Autodesk Inventor part; units mm, degrees
ref_plane "YZ Plane" through (0, 0, 0) normal (1, 0, 0) x (0, 1, 0)
ref_plane "XZ Plane" through (0, 0, 0) normal (0, 1, 0) x (-1, 0, 0)
ref_plane "XY Plane" through (0, 0, 0) normal (0, 0, 1) x (1, 0, 0)
sketch "Sketch1" plane through (0, 0, 0) normal (0, 0, 1) x (1, 0, 0)
  line L0 (-48.5, 0) -> (-48.5, 55)
  line L1 (-48.5, 55) -> (-38.5, 55)
  line L2 (-38.5, 55) -> (-38.5, 27)
  line L3 (-30.5, 19) -> (30.5, 19)
  line L4 (38.5, 27) -> (38.5, 55)
  line L5 (38.5, 55) -> (48.5, 55)
  line L6 (48.5, 55) -> (48.5, 0)
  line L7 (48.5, 0) -> (-48.5, 0)
  arc A0 (-38.5, 27) -> (-30.5, 19) centre (-30.5, 27) ccw
  arc A1 (30.5, 19) -> (38.5, 27) centre (30.5, 27) ccw
  line L8 (0, 0) -> (0, 59.4805) construction
  point P0 (0, 0)
  point P1 (0, 19)
  dimension "d0" = 10
  dimension "d1" = 19
  dimension "d2" = 36
  dimension "d3" = 8
  dimension "d4" = 97
extrude "Extrusion1" add sketch "Sketch1" against normal blind 22
sketch "Sketch2" plane through (0, 0, 0) normal (0, 0, 1) x (1, 0, 0)
  arc A0 (24.6577, 0) -> (-24.6577, 0) centre (0, -34) ccw
  line L0 (-48.5, 0) -> (48.5, 0)
  line L1 (-24.6577, 0) -> (24.6577, 0)
  point P0 (0, 0)
  point P1 (0, 0)
  point P2 (0, 0)
  point P3 (-24.6577, 0)
  point P4 (24.6577, 0)
  dimension "d7" = 84
  dimension "d8" = 8
extrude "Extrusion2" cut sketch "Sketch2" against normal up to surface (22 mm away)
sketch "Sketch3" plane through (0, 0, 0) normal (0, 0, 1) x (1, 0, 0)
  arc A0 (24.6577, 0) -> (-24.6577, 0) centre (0, -34) ccw
  line L0 (-7, 7.4126) -> (-7, 13.4126)
  line L1 (-7, 13.4126) -> (7, 13.4126)
  line L2 (7, 13.4126) -> (7, 7.4126)
  line L3 (0, 0) -> (0, 19) construction
  line L4 (30.5, 19) -> (-30.5, 19)
  dimension "d11" = 14
  dimension "d12" = 6
extrude "Extrusion3" cut sketch "Sketch3" against normal up to surface (22 mm away)
sketch "Sketch4" plane through (0, 0, 0) normal (0, 0, 1) x (1, 0, 0)
  line L0 (-48.5, 55) -> (-48.5, 0)
  line L1 (-48.5, 0) -> (-24.6577, 0)
  point P0 (0, 0)
  point P1 (-36, 16)
  dimension "d22" = 12.5
  dimension "d23" = 16
hole "Hole1" at (-36, 16, 0) direction (0, 0, -1) diameter 5.5 depth 22
sketch "Sketch5" plane through (-48.5, 0, 0) normal (-1, 0, 0) x (0, 0, 1)
  line L0 (0, 55) -> (-22, 55)
  arc A0 (-17, 55) -> (-5, 55) centre (-11, 55) ccw
  line L1 (-17, 55) -> (-5, 55)
  point P0 (0, 0)
  point P1 (-5, 55)
  dimension "d24" = 12
extrude "Extrusion4" cut sketch "Sketch5" against normal up to surface (10 mm away)
mirror "Mirror1" about plane through (0, 0, 0) normal (1, 0, 0) of "Extrusion4"
sketch "Sketch6" plane through (-48.5, 55, 0) normal (0, 1, 0) x (1, 0, 0)
  line L0 (0, 5) -> (0, 17)
  line L1 (0, 22) -> (10, 22)
  point P0 (48.5, 0)
  point P1 (5, 19)
  point P2 (5, 3)
  point P3 (0, 11)
  point P4 (5, 22)
  dimension "d27" = 8
  dimension "d28" = 8
hole "Hole2" at (-43.5, 55, -19) at (-43.5, 55, -3) direction (0, -1, 0) diameter 3 depth 5
mirror "Mirror2" about plane through (0, 0, 0) normal (1, 0, 0) of "Hole2"
fillet "Fillet1" radius 8 2 edges at (48.5, 0, -11) (-48.5, 0, -11)
sketch "Sketch7" plane through (48.5, 55, -11) normal (1, 0, 0) x (0, 0, -1)
  line L0 (-11, -55) -> (11, -55)
  point P0 (0, -42)
  point P1 (0, -55)
  dimension "d44" = 13
hole "Hole3" at (48.5, 13, -11) direction (-1, 0, 0) diameter 3.242 depth 19
sketch "Sketch8" plane through (-30.5, 19, 0) normal (0, 1, 0) x (1, 0, 0)
  line L0 (-8, 17) -> (-8, 5)
  circle A0 centre (-13, 3) radius 1.5
  circle A1 centre (-13, 19) radius 1.5
  point P0 (30.5, 0)
  point P1 (30.5, 18)
  point P2 (30.5, 4)
  point P3 (-8, 11)
  dimension "d52" = 7
  dimension "d53" = 7
  dimension "d54" = 43.5
  dimension "d55" = 43.5
hole "Hole4" at (0, 19, -18) at (0, 19, -4) direction (0, -1, 0) diameter 4 end through all
sketch "Skizze9" plane through (0, 0, 0) normal (0, 0, 1) x (1, 0, 0)
  circle A0 centre (-36, 16) radius 2.75
  arc A1 (-48.5, 8) -> (-40.5, 0) centre (-40.5, 8) ccw
  line L0 (-40.5, 0) -> (-24.6577, 0)
  arc A2 (-7, 7.4126) -> (-24.6577, 0) centre (0, -34) ccw
  line L1 (-7, 7.4126) -> (-7, 13.4126)
  line L2 (-7, 13.4126) -> (7, 13.4126)
  line L3 (7, 13.4126) -> (7, 7.4126)
  arc A3 (24.6577, 0) -> (7, 7.4126) centre (0, -34) ccw
  line L4 (24.6577, 0) -> (40.5, 0)
  arc A4 (40.5, 0) -> (48.5, 8) centre (40.5, 8) ccw
  line L5 (48.5, 8) -> (48.5, 55)
  line L6 (48.5, 55) -> (38.5, 55)
  line L7 (38.5, 55) -> (38.5, 27)
  arc A5 (30.5, 19) -> (38.5, 27) centre (30.5, 27) ccw
  line L8 (30.5, 19) -> (-30.5, 19)
  arc A6 (-38.5, 27) -> (-30.5, 19) centre (-30.5, 27) ccw
  line L9 (-38.5, 27) -> (-38.5, 55)
  line L10 (-38.5, 55) -> (-48.5, 55)
  line L11 (-48.5, 55) -> (-48.5, 8)
  arc A7 (24.6577, 0) -> (-24.6577, 0) centre (0, -34) ccw
  point P0 (0, 0)
properties part number "145 part 2" material "Aluminum 6061-AHC"
CAD build for the part. Positions are in the model's coordinates, mm. A direction names the side the tool comes from. Coordinates: 2 decimals unless noted, no trailing zeros. Loops run counter-clockwise (first coordinate to the right, second up) from the corner with the lowest first, then second, coordinate; pieces in that order, holes last. Notation, with made-up numbers: (-27.5, 2) - (-11.5, 2) arc R24 cw to (-11.5, 41) - close; hole circle Ø10 at (61, -34.5). An arc over 180 degrees is marked (long way). Return JSON: item names as keys, results as strings.
1. Band-saw the part on C-C (y = 37). Give the cut face in (x, z), and give its area (3 significant figures).
Result:
{"outline": "(-48.5, -22) - (-38.5, -22) - (-38.5, 0) - (-48.5, 0) - close; (38.5, -22) - (48.5, -22) - (48.5, 0) - (38.5, 0) - close", "area": "440 mm2"}
2. 3-axis set-ups, long thin cutter, end or side, ignore diameter. For faces 1 (the flat face through (43, 55, -21)), 2 (the cylindrical face through (-16.13, 4.78, -10.85)), 3 (the cylindrical face through (38.87, 11.9, -9.81)), 4 (the flat face through (44, 50, -3)): which of +Z, -Z, +X, -X, +Y, -Y reach the whole face in a straight line?
Result:
{"face 1": "+Z, -Z, +X, -X, +Y", "face 2": "+Z, -Z, -Y", "face 3": "+X", "face 4": "+Y"}
3. Probe L1, parallel to X at y = 53.8, z = -3; L2, parallel to Z at x = 0, y = 16.6; L3, parallel to X at y = 44.5, z = -7.5. List the from-to ranges inside material, lowest first. Write a range as from..to.
Result:
{"L1": "x = -48.5..-45, -42..-38.5, 38.5..42, 45..48.5", "L2": "z = -22..-20, -16..-6, -2..0", "L3": "x = -48.5..-38.5, 38.5..48.5"}
4. Drop flat-ended pins along their axis: pin 1 (11 mm diameter, centred on x = 15, z = -12, fed in from +Y); pin 2 (4.5 mm diameter, centred on x = -36, y = 16, fed in from +Z); pin 3 (2.5 mm diameter, centred on x = 43.5, z = -3, fed in from -Y); pin 4 (11 mm diameter, centred on x = 1, z = -14.5, fed in from -Y). Give the stop position or say it passes through.
Result:
{"pin 1": "stops at y = 19", "pin 2": "passes through", "pin 3": "stops at y = 0.19", "pin 4": "stops at y = 13.41"}
5. Band-saw the part on A-A (y = 16). Give the cut face in (x, z).
Result:
{"outline": "(-48.5, -22) - (-38.75, -22) - (-38.75, 0) - (-48.5, 0) - close; (-33.25, -22) - (48.5, -22) - (48.5, 0) - (-33.25, 0) - close; hole circle Ø4 at (0, -18); hole circle Ø4 at (0, -4)"}
6. Mould opens along Y. For faces 5 (the flat face through (-32, 0, -11)), 6 (the cylindrical face through (-38.727, 16.358, -11.154)), 7 (the flat face through (-1, 16, -22)) say: released by +Y, released by -Y, zero draft, split by the parting line, or undercut.
Result:
{"face 5": "released by -Y", "face 6": "undercut", "face 7": "zero draft"}
7. Band-saw the part on D-D (z = -7.5). Give the cut face in (x, y).
Result:
{"outline": "(-48.5, 8) arc R8 ccw to (-40.5, 0) - (-24.66, 0) arc R42 cw to (-7, 7.41) - (-7, 13.41) - (7, 13.41) - (7, 7.41) arc R42 cw to (24.66, 0) - (40.5, 0) arc R8 ccw to (48.5, 8) - (48.5, 50.13) - (38.5, 50.13) - (38.5, 27) arc R8 cw to (30.5, 19) - (-30.5, 19) arc R8 cw to (-38.5, 27) - (-38.5, 50.13) - (-48.5, 50.13) - close; hole circle Ø5.5 at (-36, 16)"}
8. Band-saw the part on B-B (x = 0). Give the cut face in (y, z), and give its area (3 significant figures).
Result:
{"outline": "(13.41, -22) - (19, -22) - (19, -20) - (13.41, -20) - close; (13.41, -16) - (19, -16) - (19, -6) - (13.41, -6) - close; (13.41, -2) - (19, -2) - (19, 0) - (13.41, 0) - close", "area": "78.2 mm2"}
